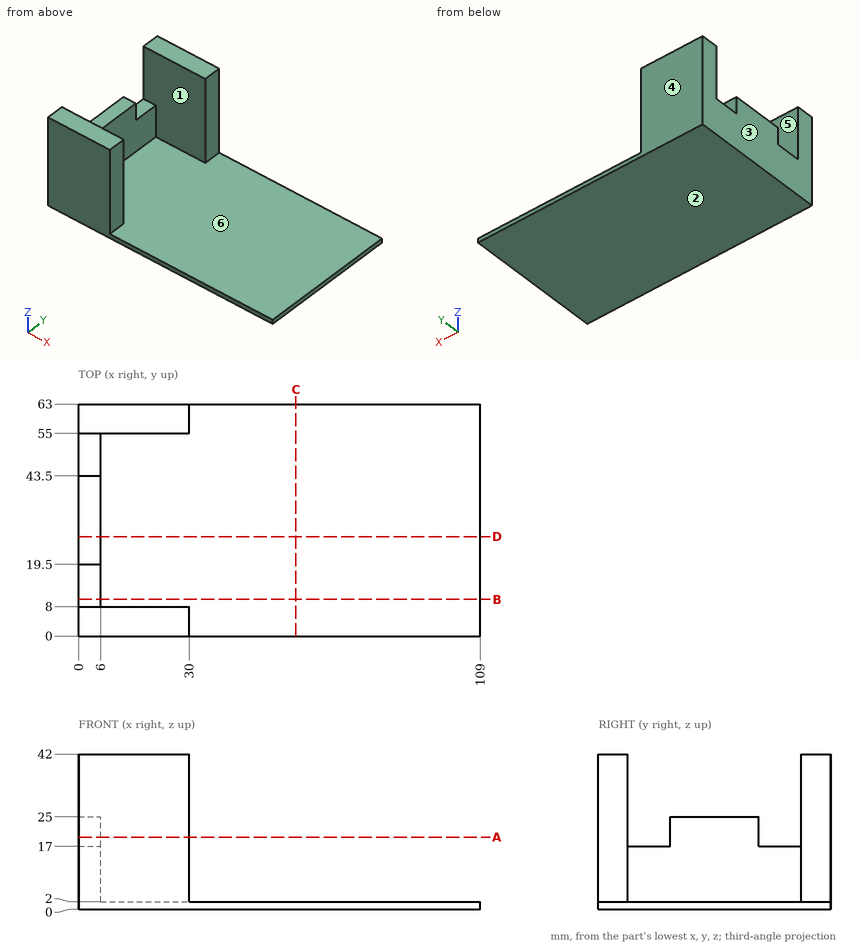
Drawing for the job (mm, zero at the part's lowest x, y, z). A direction names the side the tool comes from. Coordinates: 2 decimals unless noted, no trailing zeros. Loops run counter-clockwise (first coordinate to the right, second up) from the corner with the lowest first, then second, coordinate; pieces in that order, holes last. Notation, with made-up numbers: (62.5, 73.25) - (114.5, 73.25) arc R22 cw to (114.5, 85.25) - close; hole circle Ø6 at (5.25, -22). An arc over 180 degrees is marked (long way). Use CSV: the item, a comma, the result in double quotes. Start each with the question number.
Q1. Probe probe 1 along Y at (x, z) = (22, 10.5); probe 2 along Z at (x, y) = (17, 54); probe 3 along X at (y, z) = (47.5, 4). List the from-to ranges inside material, lowest first. Write a range as from..to.
Q2. Cut at B-B, the plane y = 10. List the corners of the cut face in (x, z).
Q3. Cut at C-C, the plane x = 59. List the corners of the cut face in (y, z).
Q4. Two-plate mould, pull along Y, no slides. Class the marked faces 3, 4, 5 and 6: +Y half, -Y half, draft (parallel to the pull), parting line (faces both ways), or undercut.
Q5. Cut at D-D, the plane y = 27. List the corners of the cut face in (x, z).
Q6. 3-axis set-ups, long thin cutter, end or side, ignore diameter. For the marked faces 1 and 2: which of +Z, -Z, +X, -X, +Y, -Y reach the whole face in a straight line?
Q7. Drop flat-ended pins along their axis: P1, Ø1.8, axis at x = 3, y = 33, coming from the +Z side; P2, Ø7, axis at y = 25, z = 19, coming from the +X side; P3, Ø19, axis at x = 36, y = 31, coming from the +Z side. Give the stop position or say it passes through.
Q8. Cut at A-A, the plane z = 19.5. List the corners of the cut face in (x, y).
Here are the results:
1,probe 1,"0..8, 55..63"
1,probe 2,"0..2"
1,probe 3,"0..6"
2,outline,"(0, 0) - (109, 0) - (109, 2) - (6, 2) - (6, 17) - (0, 17) - close"
3,outline,"(0, 0) - (63, 0) - (63, 2) - (0, 2) - close"
4,face 3,"draft"
4,face 4,"+Y half"
4,face 5,"undercut"
4,face 6,"undercut"
5,outline,"(0, 0) - (109, 0) - (109, 2) - (6, 2) - (6, 25) - (0, 25) - close"
6,face 1,"+Z, +X"
6,face 2,"-Z, +X, -X, +Y, -Y"
7,P1,"z = 25"
7,P2,"x = 6"
7,P3,"z = 2"
8,outline,"(0, 0) - (30, 0) - (30, 8) - (0, 8) - close; (0, 19.5) - (6, 19.5) - (6, 43.5) - (0, 43.5) - close; (0, 55) - (30, 55) - (30, 63) - (0, 63) - close"
